For this review, take the finished solid that the model builds, in its own axes (mm). Face numbers are marked on the shaded views. A direction names the side the tool comes from. Round coordinates to 2 decimals unless told otherwise and drop trailing zeros. Write each loop counter-clockwise with the first axis right and the second up, starting at its lowest first coordinate (ties: lowest second). Pieces come first, ordered by that corner, then holes. Notation, with made-up numbers: M -20.75,17.5 L 36.25,17.5 A21 ccw 36.25,55.5 Z; hole C 58,77 d4. An arc over 180 degrees is marked long. Use one line per item in the form item = value. Start each with the question number.
Item 1: Add section A-A (z = 0). State the section outline as (x, y) points, and give its area (3 significant figures).
Item 2: For the marked faces 1, 2, 3, 4 and 5, list the 3-axis set-ups (+Z, -Z, +X, -X, +Y, -Y) from which the entire face can be reached by the end or side of a thin tool; tool diameter is ignored.
Item 3: For line 1 (Z direction, x = 0, y = 3.25); line 2 (X direction, y = 3, z = 0); line 3 (X direction, y = 10, z = 12), list the stretches that pass through material, from the lowest coordinate up. Write a range as [from, to].
Item 4: Add section C-C (x = 1). State the section outline as (y, z) points, and give its area (3 significant figures).
Item 5: Draft analysis for pull direction Z (two halves, no side actions). For the marked faces 6, 7 and 8, state which applies: released by +Z, released by -Z, zero draft, split by the parting line, or undercut.
Item 6: For P1, Ø1, axis at y = 7, z = 6.5, coming from the +X side; P2, Ø6, axis at x = -10.5, y = 6.5, coming from the -Z side; P3, Ø3, axis at x = 18, z = -18, coming from the +Y side; P4, Ø4, axis at x = -13.5, z = 4.5, coming from the +Y side, all flat-tipped, find the tip position at first contact; note any pin that passes through.
Autodesk Inventor part; units mm, degrees
ref_plane "YZ Plane" through (0, 0, 0) normal (1, 0, 0) x (0, 1, 0)
ref_plane "XZ Plane" through (0, 0, 0) normal (0, 1, 0) x (-1, 0, 0)
ref_plane "XY Plane" through (0, 0, 0) normal (0, 0, 1) x (1, 0, 0)
sketch "Sketch1" plane through (0, 0, 0) normal (0, 1, 0) x (-1, 0, 0)
  line L0 (37.6078, 0) -> (-39.2505, 0)
  line L1 (0, -38.4978) -> (0, 39.9458)
  circle A0 centre (0, 0) radius 3.4798
  line L2 (3.1734, 25.201) -> (3.1734, 9.525)
  line L3 (-3.1734, 25.201) -> (-3.1734, 9.525)
  arc A1 (-3.1734, 9.525) -> (3.1734, 9.525) centre (0, 9.525) ccw
  line L4 (-6.35, -24.5934) -> (-6.35, -12.7)
  line L5 (6.35, -24.5934) -> (6.35, -12.7)
  arc A2 (6.35, -12.7) -> (-6.35, -12.7) centre (0, -12.7) ccw
  line L6 (-24.9495, 4.7625) -> (-11.0998, 4.7625)
  line L7 (-24.9495, -4.7625) -> (-11.0998, -4.7625)
  arc A3 (-11.0998, -4.7625) -> (-11.0998, 4.7625) centre (-11.0998, 0) ccw
  line L8 (24.1279, 7.9375) -> (14.2748, 7.9375)
  line L9 (24.1279, -7.9375) -> (14.2748, -7.9375)
  arc A4 (14.2748, 7.9375) -> (14.2748, -7.9375) centre (14.2748, 0) ccw
  arc A5 (-24.9495, -4.7625) -> (-6.35, -24.5934) centre (0, 0) ccw
  arc A6 (6.35, -24.5934) -> (24.1279, -7.9375) centre (0, 0) ccw
  arc A7 (24.1279, 7.9375) -> (3.1734, 25.201) centre (0, 0) ccw
  arc A8 (-3.1734, 25.201) -> (-24.9495, 4.7625) centre (0, 0) ccw
  dimension "d1" = 6.9596
  dimension "d5" = 9.525
  dimension "d6" = 12.7
  dimension "d7" = 9.525
  dimension "d8" = 6.3469
  dimension "d9" = 12.7
  dimension "d11" = 15.875
  dimension "d12" = 11.0998
  dimension "d13" = 14.2748
  dimension "d14" = 25.4
extrude "Extrusion1" add sketch "Sketch1" along normal blind 12.7 contours A4 L9 A6 L5 A2 L1 A0 L0 | L0 A0 L1 A1 L2 A7 L8 A4 | A0 L0 A3 L6 A8 L3 A1 L1 | L1 A2 L4 A5 L7 A3 L0 A0
chamfer "Chamfer1" distance 1.5875 angle 45 4 edges at (-16.1508, 12.7, 19.6039) (-17.3661, 12.7, -18.5359) (18.5265, 12.7, -17.3761) (17.3827, 12.7, 18.5203)
properties part number "Ch7(5) Part 3 Table"
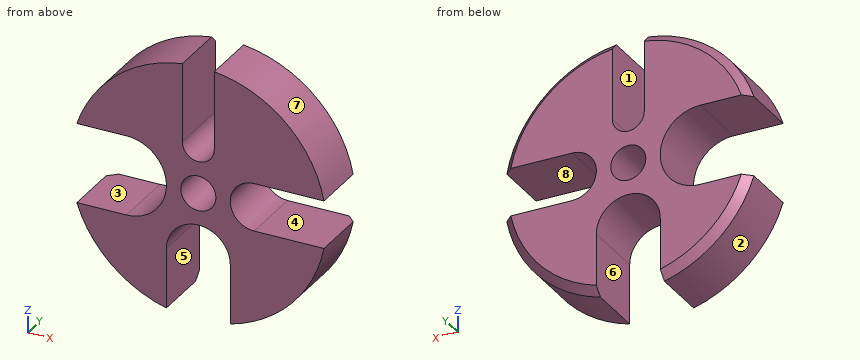
Calculated:
q1.outline = M -6.34,0 L -3.48,0 L -3.48,12.7 L -6.34,12.7 Z; M 3.48,0 L 6.34,0 L 6.34,12.7 L 3.48,12.7 Z
q1.area = 72.6 mm^2
q2.face_1 = +Z, +Y, -Y
q2.face_2 = -Z, -X, +Y, -Y
q2.face_3 = -X, +Y, -Y
q2.face_4 = +X, +Y, -Y
q2.face_5 = -Z, +Y, -Y
q3.line_1 = [-6.35, -3.48], [3.48, 6.35]
q3.line_2 = [-6.34, -3.48], [3.48, 6.34]
q3.line_3 = [-22.39, -3.17], [3.17, 22.39]
q4.outline = M 0,-6.43 L 12.7,-6.43 L 12.7,-3.33 L 0,-3.33 Z; M 0,3.33 L 12.7,3.33 L 12.7,6.51 L 0,6.51 Z
q4.area = 79.7 mm^2
q5.face_6 = zero draft
q5.face_7 = released by +Z
q5.face_8 = undercut
q6.P1 = 24.68
q6.P2 = -24.27
q6.P3 = 12.56
q6.P4 = through
